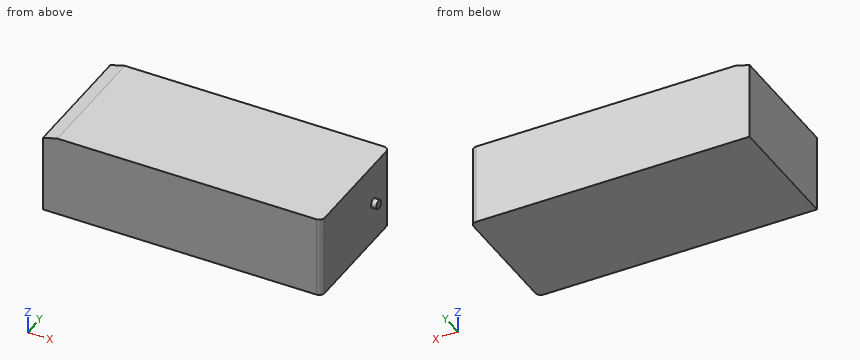
```python
from build123d import *

# Parameters (mm, degrees)
F0_W     = 51.54
F0_H     = 23.2
F1_DEPTH = 7.53
F2_R     = 1
F3_R     = 0.8075065721
F4_DEPTH = 1
F6_DEPTH = 23.2


with BuildPart() as f1:
    # F0 (on Top) → F1 (new body, symmetric)
    with BuildSketch(Plane.XY):
        Rectangle(F0_W, F0_H)
    extrude(amount=F1_DEPTH, both=True)

    # F2
    f2_edges = [f1.edges().sort_by_distance(p)[0] for p in [
        (25.77, 11.6, 0),
        (25.77, -11.6, 0),
    ]]
    fillet(f2_edges, radius=F2_R)

    # F3 (on face) → F4 (join)
    with BuildSketch(Plane.YZ.offset(25.77)):
        with Locations((6.1538815498, 0)):
            Circle(F3_R)
    extrude(amount=F4_DEPTH)

    # F5 (on face) → F6 (cut, through all)
    with BuildSketch(Plane.XZ.offset(11.6)):
        Polygon((-25.77, 7.53), (-25.77, 6.7921262234), (-23.1085941195, 7.53), align=None)
    extrude(amount=-F6_DEPTH, mode=Mode.SUBTRACT)


solid = f1.part
```
Source: CAD feature listing. Evaluate the final solid. Frame: model axes, mm. Round coordinates to 2 decimals unless told otherwise and drop trailing zeros. Loops run counter-clockwise (first coordinate to the right, second up) from the corner with the lowest first, then second, coordinate; pieces in that order, holes last.
1. Contact query for a flat-ended pin moving along its axis: pin 1 (1 mm diameter, centred on y = 1.5, z = -1.5, fed in from +X). Output: stop coordinate, or through.
2. Section query B-B on y = -6.25. Output: boundary loops of the cut face in (x, z).
3. Section query A-A on z = 0. Output: boundary loops of the cut face in (x, y).
4. Ray query, L1, parallel to X at y = -4.5, z = -4. Return the intervals inside material, ascending.
5. Section query C-C on z = -3. Output: boundary loops of the cut face in (x, y).
Answers below:
1. pin 1: stops at x = 25.77
2. outline: (-25.77, -7.53) - (25.77, -7.53) - (25.77, 7.53) - (-23.11, 7.53) - (-25.77, 6.79) - close
3. outline: (-25.77, -11.6) - (24.77, -11.6) arc R1 ccw to (25.77, -10.6) - (25.77, 5.35) - (26.77, 5.35) - (26.77, 6.96) - (25.77, 6.96) - (25.77, 10.6) arc R1 ccw to (24.77, 11.6) - (-25.77, 11.6) - close
4. L1: x = -25.77 to 25.77
5. outline: (-25.77, -11.6) - (24.77, -11.6) arc R1 ccw to (25.77, -10.6) - (25.77, 10.6) arc R1 ccw to (24.77, 11.6) - (-25.77, 11.6) - close
